Work out the finished part from the listing and answer in its coordinate system (mm). A direction names the side the tool comes from. Round coordinates to 2 decimals unless told otherwise and drop trailing zeros. Answer as a JSON object with one key per item and string values. Group by question number.
from build123d import *

# Parameters (mm, degrees)
F1_DEPTH  = 1524
F5_DEPTH  = 609.6
F11_DEPTH = 584.2
F16_R     = 71.4113893101
F17_DEPTH = 320.04


with BuildPart() as f1:
    # F0 (on Top) → F1 (new body)
    with BuildSketch(Plane.XY):
        with BuildLine():
            Line((358.775, -304.8), (301.625, -304.8))
            ThreePointArc((301.625, -304.8), (294.8898079092, -307.5898079092), (292.1, -314.325))
            Line((292.1, -314.325), (292.1, -396.875))
            ThreePointArc((292.1, -396.875), (294.8898079092, -403.6101920908), (301.625, -406.4))
            Line((301.625, -406.4), (358.775, -406.4))
            ThreePointArc((358.775, -406.4), (365.5101920908, -403.6101920908), (368.3, -396.875))
            Line((368.3, -396.875), (368.3, -314.325))
            ThreePointArc((368.3, -314.325), (365.5101920908, -307.5898079092), (358.775, -304.8))
        make_face()
        with BuildLine():
            ThreePointArc((296.8625, -314.325), (298.2574039546, -310.9574039546), (301.625, -309.5625))
            Line((301.625, -309.5625), (358.775, -309.5625))
            ThreePointArc((358.775, -309.5625), (362.1425960454, -310.9574039546), (363.5375, -314.325))
            Line((363.5375, -314.325), (363.5375, -396.875))
            ThreePointArc((363.5375, -396.875), (362.1425960454, -400.2425960454), (358.775, -401.6375))
            Line((358.775, -401.6375), (301.625, -401.6375))
            ThreePointArc((301.625, -401.6375), (298.2574039546, -400.2425960454), (296.8625, -396.875))
            Line((296.8625, -396.875), (296.8625, -314.325))
        make_face(mode=Mode.SUBTRACT)
    extrude(amount=F1_DEPTH)


with BuildPart() as f2_1:
    # F2: instance of F1
    add(f1.part.mirror(Plane.XZ))


with BuildPart() as f3_1:
    # F3: instance of F1
    add(f1.part.mirror(Plane.YZ))


with BuildPart() as f3_2:
    # F3: instance of F2_1
    add(f2_1.part.mirror(Plane.YZ))


with BuildPart() as f5:
    # F4 (on face) → F5 (new body)
    with BuildSketch(Plane.XZ.offset(-304.8)):
        Polygon((311.15, 57.15), (311.15, 50.8), (349.25, 50.8), (349.25, 127), (311.15, 127), (311.15, 120.65), (342.9, 120.65), (342.9, 57.15), align=None)
    extrude(amount=F5_DEPTH)


with BuildPart() as f7_1:
    # F7: instance of F5
    add(f5.part.mirror(Plane.XY.offset(762)))


with BuildPart() as f8_1:
    # F8: copy of F5
    add(f5.part.moved(Location((0, 0, 673.1))))


with BuildPart() as f9_1:
    # F9: instance of F8_1
    add(f8_1.part.mirror(Plane.YZ))


with BuildPart() as f9_2:
    # F9: instance of F7_1
    add(f7_1.part.mirror(Plane.YZ))


with BuildPart() as f9_3:
    # F9: instance of F5
    add(f5.part.mirror(Plane.YZ))


with BuildPart() as f11:
    # F10 (on face) → F11 (new body)
    with BuildSketch(Plane(origin=(292.1, 0, 0), x_dir=(0, -1, 0), z_dir=(-1, 0, 0))):
        Polygon((336.55, 57.15), (336.55, 50.8), (374.65, 50.8), (374.65, 127), (336.55, 127), (336.55, 120.65), (368.3, 120.65), (368.3, 57.15), align=None)
    extrude(amount=F11_DEPTH)


with BuildPart() as f12_1:
    # F12: copy of F11
    add(f11.part.moved(Location((0, 0, 762))))


with BuildPart() as f13_1:
    # F13: instance of F11
    add(f11.part.mirror(Plane.XY.offset(762)))


with BuildPart() as f1_1:
    add(f1.part)

    add(f2_1.part)  # F14 merges F2_1

    add(f3_1.part)  # F14 merges F3_1

    add(f3_2.part)  # F14 merges F3_2

    add(f5.part)  # F14 merges F5

    add(f7_1.part)  # F14 merges F7_1

    add(f8_1.part)  # F14 merges F8_1

    add(f9_1.part)  # F14 merges F9_1

    add(f9_2.part)  # F14 merges F9_2

    add(f9_3.part)  # F14 merges F9_3

    add(f11.part)  # F14 merges F11

    add(f12_1.part)  # F14 merges F12_1

    add(f13_1.part)  # F14 merges F13_1
    # F14: F11, F12_1, F13_1 across plane
    add(f11.part.mirror(Plane.XZ))
    add(f12_1.part.mirror(Plane.XZ))
    add(f13_1.part.mirror(Plane.XZ))


with BuildPart() as f17:
    # F16 (on offset) → F17 (new body)
    with BuildSketch(Plane.XZ.offset(501.65)):
        with Locations((0, 351.0118424892)):
            Circle(F16_R)
    extrude(amount=F17_DEPTH)


solid = f1_1.part
Item 1: A tool of negligible diameter and unlimited length cuts with its end or side. For faces 1 (the flat face through (330, 4, 800.1)), 2 (the flat face through (363.538, 355, 751)), 3 (the flat face through (4, -355, 1473.2)), 4 (the flat face through (331, -304.8, 751)), 5 (the flat face through (4, 355, 50.8)), from which of +Z, -Z, +X, -X, +Y, -Y can it reach the whole face along a straight path? Write none if from no direction.
Item 2: Each of these flat-tipped pins is pushed along its axis until it touches: pin 1 (16 mm diameter, centred on x = 114.5, y = -351.5, fed in from -Z); pin 2 (23 mm diameter, centred on x = 12, z = 833.5, fed in from -Y); pin 3 (1.9 mm diameter, centred on x = -50.5, z = 885.5, fed in from +Y). Where does it stop, or does it pass through?
Item 3: Find section A-A (z = 516). Give the number of separate pieces and of enclosed holes in the cut face, and give its area (3 significant figures).
Item 4: Consider L1, parallel to Y at x = 309, z = 222; L2, parallel to X at y = -323, z = 1131.5; L3, parallel to Y at x = -136.5, z = 816. Determine where each line is inside the solid, lowest interval first.
Item 5: The mould has two halves that part along X. Classify faces 6 (the flat face through (-363.538, -355, 751)), 7 (the flat face through (-330, 4, 800.1)): +X half, -X half, draft (parallel to the pull), parting line (faces both ways), or undercut.
Responses:
{
 "1": {"face 1": "+X, -X", "face 2": "+Z, -Z", "face 3": "+Z, +Y, -Y", "face 4": "none", "face 5": "-Z, +Y, -Y"},
 "2": {"pin 1": "stops at z = 50.8", "pin 2": "stops at y = -374.65", "pin 3": "stops at y = 374.65"},
 "3": {"separate pieces": "4", "enclosed holes": "4", "area": "6,180 mm^2"},
 "4": {"L1": "y = -406.4 to -401.64, -309.56 to -304.8, 304.8 to 309.56, 401.64 to 406.4", "L2": "x = -368.3 to -363.54, -296.86 to -292.1, 292.1 to 296.86, 363.54 to 368.3", "L3": "y = -374.65 to -336.55, 336.55 to 374.65"},
 "5": {"face 6": "undercut", "face 7": "draft"}
}
